CAD build for the part. Positions are in the model's coordinates, mm. Round coordinates to 2 decimals unless told otherwise and drop trailing zeros. Loops run counter-clockwise (first coordinate to the right, second up) from the corner with the lowest first, then second, coordinate; pieces in that order, holes last.
from build123d import *

# Parameters (mm, degrees)
SWEEP1_PROFILE_R        = 12.5
SKETCH6_R               = 5
CUT_EXTRUDE1_DEPTH      = 13.5
CUT_EXTRUDE1_DEPTH_BACK = 13.5
FILLET1_R               = 0.5


with BuildPart() as part:
    # Sweep1: sweep along a path in Sketch1
    with BuildLine(Plane.XY) as sweep1_path:
        Line((0, 0), (0, 152.4))
    # Sweep1 profile (on start of the path) → Sweep1 (sweep)
    with BuildSketch(Plane.ZX):
        Circle(SWEEP1_PROFILE_R)
    sweep(path=sweep1_path.line)

    # Sketch6 → Cut-Extrude1 (cut, two sides)
    with BuildSketch(Plane.XY) as cut_extrude1_sk:
        with Locations((0, 139.9)):
            Circle(SKETCH6_R)
    extrude(amount=CUT_EXTRUDE1_DEPTH, mode=Mode.SUBTRACT)
    extrude(cut_extrude1_sk.sketch, amount=-CUT_EXTRUDE1_DEPTH_BACK, mode=Mode.SUBTRACT)

    # Fillet1
    fillet1_edges = [part.edges().sort_by_distance(p)[0] for p in [
        (0, 0, -12.5),
        (0, 152.4, -12.5),
    ]]
    fillet(fillet1_edges, radius=FILLET1_R)


solid = part.part
Item 1: Wall check: L1, parallel to Y at x = -0.5, z = 0.5; L2, parallel to Y at x = -2.25, z = -5.5; L3, parallel to Z at x = -0.25, y = 113. Give the ranges that are in metal, low to high.
Verdict:
L1: y = 0 to 134.93, 144.87 to 152.4
L2: y = 0 to 135.43, 144.37 to 152.4
L3: z = -12.5 to 12.5
Item 2: Cut at A-A (x = 0). List the corners of the cut face in (y, z), plus the area to 3 significant figures.
Verdict:
outline: (0, -12) arc R0.5 ccw to (0.5, -12.5) - (134.9, -12.5) - (134.9, 12.5) - (0.5, 12.5) arc R0.5 ccw to (0, 12) - close; (144.9, -12.5) - (151.9, -12.5) arc R0.5 ccw to (152.4, -12) - (152.4, 12) arc R0.5 ccw to (151.9, 12.5) - (144.9, 12.5) - close
area: 3,560 mm2
Item 3: Flat gauge pins, fed straight in: P1, Ø6, axis at y = 47.5, z = -3, coming from the +X side; P2, Ø12, axis at x = -7.5, y = 94.5, coming from the +Z side; P3, Ø1.5, axis at y = 119, z = -9, coming from the +X side; P4, Ø4, axis at y = 71, z = -6, coming from the -X side. Where does each tip first touch, or does it go through?
Verdict:
P1: stops at x = 12.5
P2: stops at z = 12.41
P3: stops at x = 9.39
P4: stops at x = -11.84
Item 4: Cut at B-B (y = 26). List the corners of the cut face in (x, z), plus the area to 3 significant figures.
Verdict:
outline: circle Ø25 at (0, 0)
area: 491 mm2
